The model under review builds one solid part; all positions refer to its coordinate system, in mm. Face numbers are marked on the shaded views. A direction names the side the tool comes from. Round coordinates to 2 decimals unless told otherwise and drop trailing zeros. Order: outer loops, then holes, each group sorted by start corner. A loop starts at its lowest first (then second) coordinate and runs counter-clockwise, first axis right, second up. Notation, with made-up numbers: (64.5, -2.75) -> (108.5, -2.75) arc R20 ccw to (108.5, 24.25) -> close; hole circle Ø4 at (18, 67). An arc over 180 degrees is marked (long way). Use a Markdown table: item, result. Add a question column.
```python
from build123d import *

# Parameters (mm, degrees)
Y_KSEKLIK_EKSTR_ZYON1_DEPTH = 3.75
IZIM2_R                     = 1.25
Y_KSEKLIK_EKSTR_ZYON2_DEPTH = 30
IZIM3_OUTSIDE_W             = 63.452
IZIM3_OUTSIDE_H             = 60.976
IZIM3_OUTSIDE_R             = 8
KES_EKSTR_ZYON1_DEPTH       = 10
KES_EKSTR_ZYON1_DRAFT       = -60
IZIM4_OUTSIDE_W             = 63.452
IZIM4_OUTSIDE_H             = 60.976
IZIM4_OUTSIDE_R             = 8
KES_EKSTR_ZYON2_DEPTH       = 10
KES_EKSTR_ZYON2_DRAFT       = -60


with BuildPart() as part:
    # Çizim1 → Yükseklik-Ekstrüzyon1 (new body)
    with BuildSketch(Plane(origin=(0, 0, 0), x_dir=(0, 0, -1), z_dir=(1, 0, 0))):
        Polygon((-6.225342033, 7.865351493), (-10.844144187, 15.865351493), (-20.081748494, 15.865351493), (-24.700550647, 7.865351493), (-20.081748494, -0.134648507), (-10.844144187, -0.134648507), align=None)
    extrude(amount=Y_KSEKLIK_EKSTR_ZYON1_DEPTH)

    # Çizim2 → Yükseklik-Ekstrüzyon2 (add)
    with BuildSketch(Plane(origin=(3.75, 0, 0), x_dir=(0, 0, -1), z_dir=(1, 0, 0))):
        with Locations((-15.46294634, 7.865351493)):
            Circle(IZIM2_R)
    extrude(amount=Y_KSEKLIK_EKSTR_ZYON2_DEPTH)


with BuildPart() as kes_ekstr_zyon1_tool:
    # Çizim3 outside → Kes-Ekstrüzyon1 (with draft: the straight prism first)
    with BuildSketch(Plane.ZY):
        with Locations((15.463, 7.865)):
            Rectangle(IZIM3_OUTSIDE_W, IZIM3_OUTSIDE_H)
        with Locations((15.46294634, 7.865351493)):
            Circle(IZIM3_OUTSIDE_R, mode=Mode.SUBTRACT)
    extrude(amount=-KES_EKSTR_ZYON1_DEPTH)
    # Kes-Ekstrüzyon1: the draft: its side faces are tilted about the plane it starts from
    kes_ekstr_zyon1_sides = [kes_ekstr_zyon1_tool.faces().sort_by_distance(p)[0] for p in [
        (5, -22.623, 15.463),
        (5, 7.865, 47.189),
        (5, 38.353, 15.463),
        (5, 7.865, -16.263),
        (5, 7.865351493, 7.46294634),
    ]]
    draft(kes_ekstr_zyon1_sides, Plane.ZY, KES_EKSTR_ZYON1_DRAFT)


with BuildPart() as part_1:
    add(part.part)

    # Kes-Ekstrüzyon1: cut by kes_ekstr_zyon1_tool
    add(kes_ekstr_zyon1_tool.part, mode=Mode.SUBTRACT)


with BuildPart() as kes_ekstr_zyon2_tool:
    # Çizim4 outside → Kes-Ekstrüzyon2 (with draft: the straight prism first)
    with BuildSketch(Plane(origin=(3.75, 0, 0), x_dir=(0, 0, -1), z_dir=(1, 0, 0))):
        with Locations((-15.463, 7.865)):
            Rectangle(IZIM4_OUTSIDE_W, IZIM4_OUTSIDE_H)
        with Locations((-15.46294634, 7.865351493)):
            Circle(IZIM4_OUTSIDE_R, mode=Mode.SUBTRACT)
    extrude(amount=-KES_EKSTR_ZYON2_DEPTH)
    # Kes-Ekstrüzyon2: the draft: its side faces are tilted about the plane it starts from
    kes_ekstr_zyon2_sides = [kes_ekstr_zyon2_tool.faces().sort_by_distance(p)[0] for p in [
        (-1.25, -22.623, 15.463),
        (-1.25, 7.865, -16.263),
        (-1.25, 38.353, 15.463),
        (-1.25, 7.865, 47.189),
        (-1.25, 7.865351493, 23.46294634),
    ]]
    draft(kes_ekstr_zyon2_sides, Plane(origin=(3.75, 0, 0), x_dir=(0, 0, -1), z_dir=(1, 0, 0)), KES_EKSTR_ZYON2_DRAFT)


with BuildPart() as part_2:
    add(part_1.part)

    # Kes-Ekstrüzyon2: cut by kes_ekstr_zyon2_tool
    add(kes_ekstr_zyon2_tool.part, mode=Mode.SUBTRACT)


solid = part_2.part
```
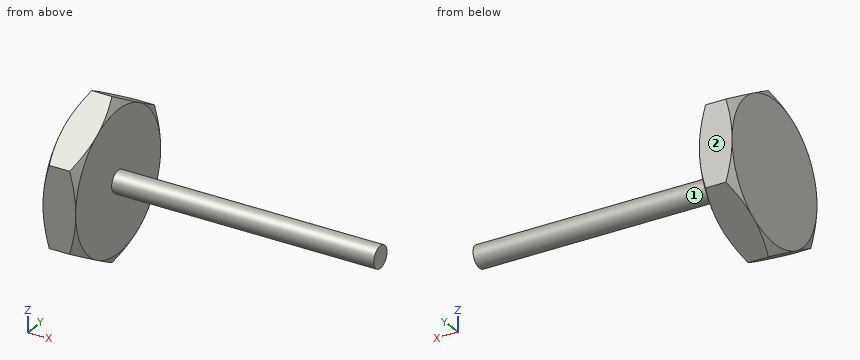
Q1. Add section A-A (x = 16.5). Write out the cut boundary in (y, z), then the cut area to 3 significant figures.
Q2. Insertion check: pin 1 (3 mm diameter, centred on x = 25.5, z = 18.5, fed in from -Y); pin 2 (4 mm diameter, centred on y = 7, z = 19, fed in from +X); pin 3 (5 mm diameter, centred on x = 19, y = 6.5, fed in from +Z). Each pin has a flat end and moves straight along its axis. Give the tip position at first contact, or say it passes through.
Q3. Wall thickness on line 1 (X direction, y = 11.75, z = 13.75); line 2 (Z direction, x = 22, y = 8); line 3 (X direction, y = 9.5, z = 7.25): over which ranges is each line inside the solid? List them lowest first. Write a range as [from, to].
Q4. Machinability: for the marked faces 1 and 2, which of the approach directions +Z, -Z, +X, -X, +Y, -Y give a long, thin tool a straight path to every point of the face, cutting with its end or side? Answer none if there is none.
Report:
| question | item | result |
|---|---|---|
| 1 | outline | circle Ø2.5 at (7.87, 15.46) |
| 1 | area | 4.91 mm² |
| 2 | pin 1 | passes through |
| 2 | pin 2 | stops at x = 3.75 |
| 2 | pin 3 | stops at z = 16.71 |
| 3 | line 1 | x = [0, 3.75] |
| 3 | line 2 | z = [14.22, 16.71] |
| 3 | line 3 | x = [0.22, 3.53] |
| 4 | face 1 | +X |
| 4 | face 2 | +Z, -Z, +X, -X, +Y |
